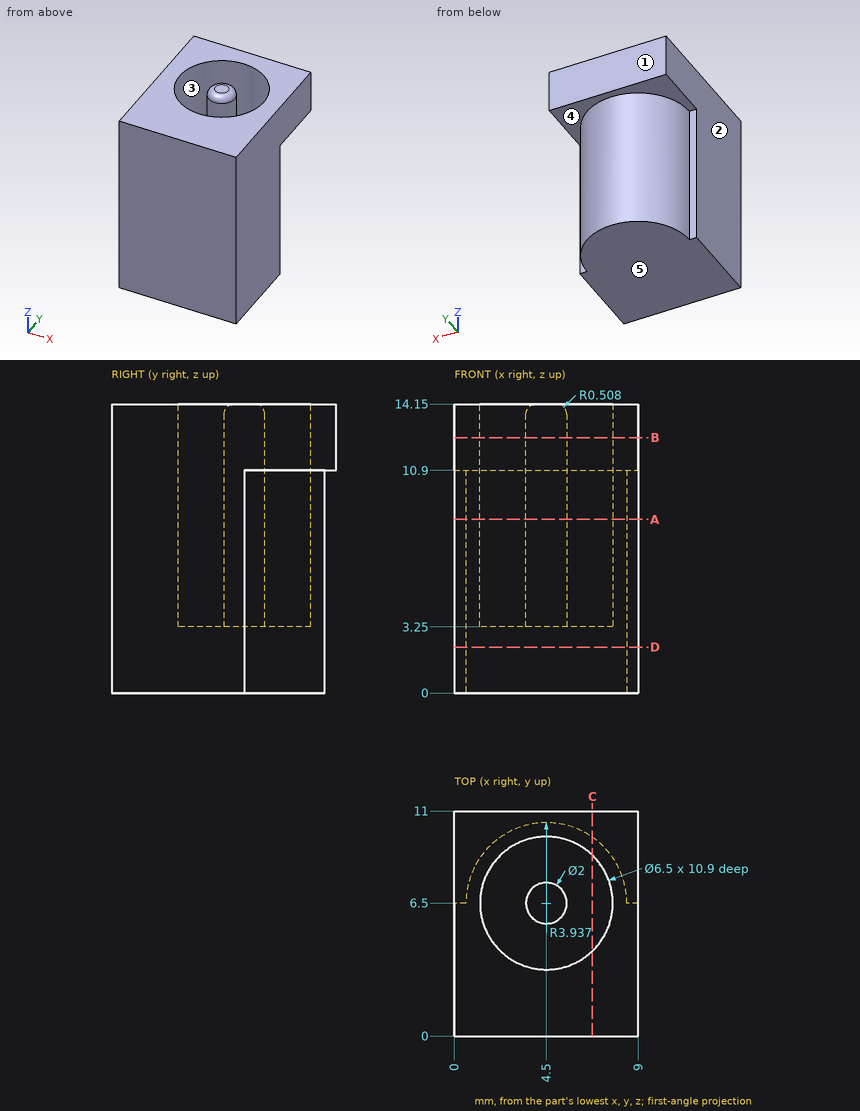
Could you check a few things on this drawing? It's one solid part, dimensions in mm from its lowest x, y, z. A direction names the side the tool comes from. Give positions to 0.01 mm unless a question says otherwise; leave off trailing zeros. Order: outer loops, then holes, each group sorted by start corner. A loop starts at its lowest first (then second) coordinate and runs counter-clockwise, first axis right, second up. Notation, with made-up numbers: (78, 19.5) - (84, 19.5) arc R25 cw to (84, 36.5) - close; hole circle Ø6 at (-39, 81.5). An arc over 180 degrees is marked (long way). Answer as a JSON object with one key per item and string values. Group by question number.
Item 1: Please list where these lines run through material, in increasing order: probe 1 along Y at (x, z) = (4.5, 10.25); probe 2 along Y at (x, z) = (4.5, 11.25); probe 3 along Z at (x, y) = (5.75, 5.25).
Item 2: If we mould it in two halves opening along X, with no side actions, what happens to the marked faces 1, 2 and 3? For each: pulls with the +X half, pulls with the -X half, needs draft (parallel to the pull), parting line crosses it, or undercut.
Item 3: Which directions (+Z, -Z, +X, -X, +Y, -Y) give clear straight access to the entire face, cutting with the end or side of a thin tool? Please do the marked faces 4 and 5.
Item 4: If we section it at C-C on x = 6.75: Please give me the cut outline in (y, z), and give its area (3 significant figures).
Item 5: If we section it at D-D on z = 2.25: Please give me the cut outline in (x, y), and give its area (3 significant figures).
Item 6: If we section it at B-B on z = 12.5: Please give me the cut outline in (x, y).
Item 7: If we section it at A-A on z = 8.5: Please give me the cut outline in (x, y).
Result set:
{
 "1": {"probe 1": "0 to 3.25, 5.5 to 7.5, 9.75 to 10.44", "probe 2": "0 to 3.25, 5.5 to 7.5, 9.75 to 11", "probe 3": "0 to 3.25"},
 "2": {"face 1": "needs draft", "face 2": "pulls with the -X half", "face 3": "undercut"},
 "3": {"face 4": "-Z, +Y", "face 5": "-Z, +X, -X, +Y, -Y"},
 "4": {"outline": "(0, 0) - (9.73, 0) - (9.73, 10.9) - (11, 10.9) - (11, 14.15) - (8.85, 14.15) - (8.85, 3.25) - (4.15, 3.25) - (4.15, 14.15) - (0, 14.15) - close", "area": "90.7 mm²"},
 "5": {"outline": "(0, 0) - (9, 0) - (9, 6.5) - (8.44, 6.5) arc R3.94 ccw to (0.56, 6.5) - (0, 6.5) - close", "area": "82.8 mm²"},
 "6": {"outline": "(0, 0) - (9, 0) - (9, 11) - (0, 11) - close; circle Ø2 at (4.5, 6.5); hole circle Ø6.5 at (4.5, 6.5)"},
 "7": {"outline": "(0, 0) - (9, 0) - (9, 6.5) - (8.44, 6.5) arc R3.94 ccw to (0.56, 6.5) - (0, 6.5) - close; circle Ø2 at (4.5, 6.5); hole circle Ø6.5 at (4.5, 6.5)"}
}
